Geometry: final body of the model. Coordinates: model frame, mm. Give positions to 0.01 mm unless a question says otherwise; leave off trailing zeros. Loops run counter-clockwise (first coordinate to the right, second up) from the corner with the lowest first, then second, coordinate; pieces in that order, holes last. Notation, with made-up numbers: (11, -18.5) -> (52, -18.5) arc R30 cw to (52, 5.5) -> close; hole circle Ø9 at (-12, 31.25). An arc over 180 degrees is marked (long way). One line per question, with ' | ' between items. Start each with the question number.
Item 1: Material intervals for line 1 along Y through (x, z) = (-0.35, 35), sorted ascending. Write a range as [from, to].
Item 2: Section A-A on x = -1.8. Return loops of the section in (y, z), then the cut area to 3 significant figures.
Item 3: Section B-B on z = 37. Return loops of the section in (x, y).
Item 4: Pin query (flat end, axial travel): P1, Ø0.9, axis at x = -2, z = 29.5, coming from the +Y side. Return the tip coordinate at first contact, or that it passes through.
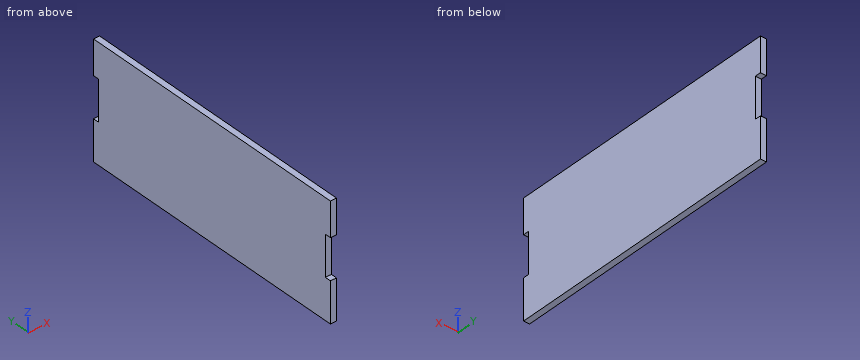
Autodesk Inventor part; units mm, degrees
ref_plane "YZ Plane" through (0, 0, 0) normal (1, 0, 0) x (0, 1, 0)
ref_plane "XZ Plane" through (0, 0, 0) normal (0, 1, 0) x (-1, 0, 0)
ref_plane "XY Plane" through (0, 0, 0) normal (0, 0, 1) x (1, 0, 0)
sketch "Sketch1" plane through (0, 0, 0) normal (1, 0, 0) x (0, 1, 0)
  line L0 (0, 0) -> (0, 20)
  line L1 (0, 0) -> (-70, 0)
  line L2 (-70, 0) -> (-70, 57)
  line L3 (-70, 57) -> (0, 57)
  line L4 (0, 57) -> (0, 0)
  line L5 (0, 0) -> (-3, 0)
  line L6 (-3, 0) -> (-3, 20)
  line L7 (-3, 20) -> (0, 20)
  line L8 (0, 20) -> (0, 0)
  line L9 (-3, 20) -> (0, 20)
  line L10 (0, 20) -> (0, 40)
  line L11 (0, 40) -> (-3, 40)
  line L12 (-3, 40) -> (-3, 20)
  line L13 (-3, 40) -> (-3, 57)
  line L14 (0, 40) -> (0, 57)
  dimension "d0" = 20
  dimension "d1" = 70
  dimension "d2" = 57
  dimension "d3" = 3
  dimension "d4" = 20
  dimension "d5" = 3
  dimension "d6" = 20
extrude "Extrusion1" add sketch "Sketch1" against normal blind 3 contours L1 L6 L7 L0 | L1 L2 L3 L13 L12 L6 | L11 L13 L3 L4
mirror "Mirror1" about plane through (0, -70, 0) normal (0, -1, 0) of "Extrusion1"
properties part number "dak"
Result sheet:
1) line 1: y = [-137, -3]
2) outline: (-140, 0) -> (0, 0) -> (0, 20) -> (-3, 20) -> (-3, 40) -> (0, 40) -> (0, 57) -> (-140, 57) -> (-140, 40) -> (-137, 40) -> (-137, 20) -> (-140, 20) -> close | area: 7,860 mm²
3) outline: (-3, -137) -> (0, -137) -> (0, -3) -> (-3, -3) -> close
4) P1: stops at y = -3
